Geometry: final body of the model. Coordinates: model frame, mm. A direction names the side the tool comes from. Round coordinates to 2 decimals unless told otherwise and drop trailing zeros. Order: outer loops, then holes, each group sorted by start corner. A loop starts at its lowest first (then second) coordinate and runs counter-clockwise, first axis right, second up. Notation, with made-up numbers: M 70.5,83.25 L 86.5,83.25 A17 cw 86.5,92.25 Z; hole C 38.5,67.5 d8. An arc over 180 degrees is marked long. Put each result on its own line as item: value. Start each with the question number.
1) Section A-A, the plane x = 0. Return loops of the section in (y, z).
2) Draft query along X for faces 4 (the flat face through (-14.98, 6.07, -26.017)), 5 (the flat face through (16, 11, 22)), 6 (the flat face through (8.23, 5.58, -28.42)). Return one class per face: pulls with the +X half, pulls with the -X half, needs draft (parallel to the pull), parting line crosses it, or undercut.
3) Section C-C, the plane x = -36. Return loops of the section in (y, z).
4) Section B-B, the plane z = 0. Count the separate pieces of the cut face and the enclosed holes in it, then the cut area to 3 significant figures.
5) First-contact query: P1, Ø7, axis at x = 18.01, z = 31.2, coming from the -Y side; P2, Ø4, axis at x = -12, y = 6.5, coming from the +Z side; P3, Ø6, axis at y = 8.5, z = 16.5, coming from the +X side. Flat tips, straight axial feed; report the tip coordinate or a pass-through.
6) Access query for faces 1 (the cylindrical face through (31.626, 2.662, -0.193)), 2 (the flat face through (21, 6, 21.338)), 3 (the flat face through (8.03, 0.49, -18.91)). Directions: +Z, -Z, +X, -X, +Y, -Y. A direction counts if a zero-diameter tool reaches every point of the face in a straight line with its end or side. Return the directions, or none.
7) Material intervals for probe 1 along Z at (x, y) = (0, 4.25); probe 2 along X at (y, z) = (4.35, 0); probe 3 along X at (y, z) = (7.25, 29), sorted ascending. Write a range as [from, to].
from build123d import *

# Parameters (mm, degrees)
SKETCH2_R               = 42.5
BOSS_EXTRUDE1_DEPTH     = 11
CUT_EXTRUDE3_DEPTH      = 11
SKETCH4_R               = 2.65
CUT_EXTRUDE4_DEPTH      = 12
SKETCH7_W               = 20
SKETCH7_H               = 5
BOSS_EXTRUDE2_DEPTH     = 1
SKETCH6_R               = 4.4
CUT_EXTRUDE6_DEPTH      = 5.4
SKETCH8_R               = 7.5
CUT_EXTRUDE7_DEPTH      = 1
CUT_EXTRUDE7_DEPTH_BACK = 12
BOSS_EXTRUDE3_DEPTH     = 1
CIRPATTERN1_COUNT       = 6


with BuildPart() as part:
    # Sketch2 → Boss-Extrude1 (new body)
    with BuildSketch(Plane(origin=(0, 0, 0), x_dir=(1, 0, 0), z_dir=(0, 1, 0))):
        Circle(SKETCH2_R)
    extrude(amount=BOSS_EXTRUDE1_DEPTH)

    # Sketch3 → Cut-Extrude3 (cut)
    with BuildSketch(Plane(origin=(0, 11, 0), x_dir=(1, 0, 0), z_dir=(0, 1, 0))):
        Polygon((10.876265015, 23.838243603), (5.505548638, 33.14059724), (-5.505548638, 33.14059724), (-10.876265015, 23.838243602), (-12.845675931, 27.249363369), (-17.175802949, 24.749363369), (-15.206392034, 21.338243603), (-25.947824787, 21.338243602), (-31.453373426, 11.802353637), (-26.082657049, 2.5), (-30.02147888, 2.5), (-30.02147888, -2.5), (-26.082657049, -2.5), (-31.453373426, -11.802353638), (-25.947824787, -21.338243603), (-15.206392034, -21.338243603), (-17.175802949, -24.749363369), (-12.845675931, -27.249363369), (-10.876265015, -23.838243603), (-5.505548638, -33.14059724), (5.505548638, -33.14059724), (10.876265015, -23.838243602), (12.845675931, -27.249363369), (17.175802949, -24.749363369), (15.206392034, -21.338243603), (25.947824787, -21.338243602), (31.453373426, -11.802353637), (26.082657049, -2.5), (30.02147888, -2.5), (30.02147888, 2.5), (26.082657049, 2.5), (31.453373426, 11.802353637), (25.947824787, 21.338243602), (15.206392034, 21.338243602), (17.175802949, 24.749363369), (12.845675931, 27.249363369), align=None)
        Polygon((-5.235884115, 14.06881731), (5.235884115, 14.06881731), (2.845675931, 9.928855294), (7.175802949, 7.428855294), (9.566011134, 11.56881731), (14.801895249, 2.5), (10.02147888, 2.5), (10.02147888, -2.5), (14.801895249, -2.5), (9.566011134, -11.56881731), (7.175802949, -7.428855294), (2.845675931, -9.928855294), (5.235884115, -14.06881731), (-5.235884115, -14.06881731), (-2.845675931, -9.928855294), (-7.175802949, -7.428855294), (-9.566011134, -11.56881731), (-14.801895249, -2.5), (-10.02147888, -2.5), (-10.02147888, 2.5), (-14.801895249, 2.5), (-9.566011134, 11.56881731), (-7.175802949, 7.428855294), (-2.845675931, 9.928855294), align=None, mode=Mode.SUBTRACT)
    extrude(amount=-CUT_EXTRUDE3_DEPTH, mode=Mode.SUBTRACT)

    # Sketch4 → Cut-Extrude4 (cut, through all)
    with BuildSketch(Plane(origin=(0, 11, 0), x_dir=(1, 0, 0), z_dir=(0, 1, 0))):
        with Locations((18.01073944, 31.195515792)):
            Circle(SKETCH4_R)
        with Locations((36.02147888, 0)):
            Circle(SKETCH4_R)
        with Locations((18.01073944, -31.195515792)):
            Circle(SKETCH4_R)
        with Locations((-18.01073944, -31.195515792)):
            Circle(SKETCH4_R)
        with Locations((-36.02147888, 0)):
            Circle(SKETCH4_R)
        with Locations((-18.01073944, 31.195515792)):
            Circle(SKETCH4_R)
    extrude(amount=-CUT_EXTRUDE4_DEPTH, mode=Mode.SUBTRACT)

    # Sketch7 → Boss-Extrude2 (add)
    with BuildSketch(Plane.XZ):
        Polygon((-7.175802949, 7.428855294), (-2.845675931, 9.928855294), (-12.845675931, 27.249363369), (-17.175802949, 24.749363369), align=None)
        Polygon((12.845675931, 27.249363369), (2.845675931, 9.928855294), (7.175802949, 7.428855294), (17.175802949, 24.749363369), align=None)
        with Locations((20.02147888, 0)):
            Rectangle(SKETCH7_W, SKETCH7_H)
        Polygon((17.175802949, -24.749363369), (7.175802949, -7.428855294), (2.845675931, -9.928855294), (12.845675931, -27.249363369), align=None)
        Polygon((-12.845675931, -27.249363369), (-2.845675931, -9.928855294), (-7.175802949, -7.428855294), (-17.175802949, -24.749363369), align=None)
        with Locations((-20.02147888, 0)):
            Rectangle(SKETCH7_W, SKETCH7_H)
    extrude(amount=-BOSS_EXTRUDE2_DEPTH)

    # Sketch6 → Cut-Extrude6 (cut)
    with BuildSketch(Plane(origin=(0, 0, 0), x_dir=(1, 0, 0), z_dir=(0, 1, 0))):
        with Locations((18.01073944, 31.195515792)):
            Circle(SKETCH6_R)
        with Locations((36.02147888, 0)):
            Circle(SKETCH6_R)
        with Locations((18.01073944, -31.195515792)):
            Circle(SKETCH6_R)
        with Locations((-18.01073944, -31.195515792)):
            Circle(SKETCH6_R)
        with Locations((-36.02147888, 0)):
            Circle(SKETCH6_R)
        with Locations((-18.01073944, 31.195515792)):
            Circle(SKETCH6_R)
    extrude(amount=CUT_EXTRUDE6_DEPTH, mode=Mode.SUBTRACT)

    # Sketch8 → Cut-Extrude7 (cut, two sides)
    with BuildSketch(Plane(origin=(0, 11, 0), x_dir=(1, 0, 0), z_dir=(0, 1, 0))) as cut_extrude7_sk:
        Circle(SKETCH8_R)
    extrude(amount=CUT_EXTRUDE7_DEPTH, mode=Mode.SUBTRACT)
    extrude(cut_extrude7_sk.sketch, amount=-CUT_EXTRUDE7_DEPTH_BACK, mode=Mode.SUBTRACT)

    # Sketch11 → Boss-Extrude3 (add)
    with BuildSketch(Plane.XZ):
        Polygon((17.206392034, 21.338243603), (14.206392034, 19.606192795), (15.206392034, 21.338243603), align=None)
        Polygon((25.947824787, 21.338243602), (26.947824787, 19.606192795), (23.947824787, 21.338243603), align=None)
        Polygon((30.453373426, 10.07030283), (31.453373426, 11.802353637), (30.453373426, 13.534404445), align=None)
        Polygon((24.082657049, 2.5), (27.082657049, 4.232050808), (26.082657049, 2.5), align=None)
        Polygon((13.801895249, 4.232050808), (14.801895249, 2.5), (16.801895249, 2.5), align=None)
        Polygon((10.566011134, 9.836766502), (9.566011134, 11.56881731), (10.566011134, 13.300868118), align=None)
    boss_extrude3 = extrude(amount=-BOSS_EXTRUDE3_DEPTH)

    # CirPattern1: Boss-Extrude3 ×6 about axis
    cirpattern1_axis = Axis((0, 0, 0), (0, 1, 0))
    for i in range(1, CIRPATTERN1_COUNT):
        add(boss_extrude3.rotate(cirpattern1_axis, i * 360 / CIRPATTERN1_COUNT))


solid = part.part
Result sheet:
1. outline: M 0,-42.5 L 11,-42.5 L 11,-33.14 L 0,-33.14 Z; M 0,-14.07 L 11,-14.07 L 11,-7.5 L 0,-7.5 Z; M 0,7.5 L 11,7.5 L 11,14.07 L 0,14.07 Z; M 0,33.14 L 11,33.14 L 11,42.5 L 0,42.5 Z
2. face 4: undercut
2. face 5: needs draft
2. face 6: undercut
3. outline: M 0,-22.59 L 11,-22.59 L 11,-2.65 L 5.4,-2.65 L 5.4,-4.4 L 0,-4.4 Z; M 0,4.4 L 5.4,4.4 L 5.4,2.65 L 11,2.65 L 11,22.59 L 0,22.59 Z
4. separate pieces: 4
4. enclosed holes: 0
4. area: 216 mm2
5. P1: stops at y = 5.4
5. P2: stops at z = 41.31
5. P3: stops at x = 40.3
6. face 1: -Y
6. face 2: +Y
6. face 3: +Y, -Y
7. probe 1: z = [-42.5, -33.14], [-14.07, -7.5], [7.5, 14.07], [33.14, 42.5]
7. probe 2: x = [-42.5, -40.42], [-31.62, -30.02], [-10.02, -7.5], [7.5, 10.02], [30.02, 31.62], [40.42, 42.5]
7. probe 3: x = [-31.07, -19.49], [-16.53, -7.9], [7.9, 16.53], [19.49, 31.07]
